from build123d import *

# Parameters (mm, degrees)
SKETCH1_R                                    = 10
BOSS_EXTRUDE1_DEPTH                          = 6
CBORE_FOR_M3_HEX_SOCKET_HEAD_CAP_SCR_2_COUNT = 2
CBORE_FOR_M3_HEX_SOCKET_HEAD_CAP_SCR_2_PITCH = 9.192388155
CBORE_FOR_M3_HEX_SOCKET_HEAD_CAP_SCR_3_COUNT = 2
CBORE_FOR_M3_HEX_SOCKET_HEAD_CAP_SCR_3_PITCH = 13
BOSS_EXTRUDE2_START                          = -6
SKETCH6_W                                    = 120
SKETCH6_H                                    = 40
SKETCH6_R                                    = 10
BOSS_EXTRUDE2_DEPTH                          = 6


# Read off the part's stored shape, not the designer's step: Tap Drill for M4 Helicoil1
with BuildPart() as part:
    # Sketch1 → Boss-Extrude1 (new body)
    with BuildSketch(Plane.XY):
        Circle(SKETCH1_R)
    extrude(amount=BOSS_EXTRUDE1_DEPTH)

    # Sketch5 → CBORE for M3 Hex Socket Head Cap Screw1 (revolve, cut)
    with BuildSketch(Plane(origin=(-6.5, 0, 6), x_dir=(0, -1, 0), z_dir=(1, 0, 0))):
        Polygon((0, 0), (0, 6), (1.7, 6), (1.7, 3.4), (3.25, 3.4), (3.25, 0.025), (3.275, 0), align=None)
    cbore_for_m3_hex_socket_head_cap_screw1 = revolve(axis=Axis((-6.5, 0, 12.35), (0, 0, -1)), mode=Mode.SUBTRACT)

    # CBORE for M3 Hex Socket Head Cap Scr 2: CBORE for M3 Hex Socket Head Cap Screw1 ×2
    with Locations(*[Vector(0.7071067811865476, 0.7071067811865476, 0) * (i * CBORE_FOR_M3_HEX_SOCKET_HEAD_CAP_SCR_2_PITCH) for i in range(1, CBORE_FOR_M3_HEX_SOCKET_HEAD_CAP_SCR_2_COUNT)]):
        add(cbore_for_m3_hex_socket_head_cap_screw1, mode=Mode.SUBTRACT)

    # CBORE for M3 Hex Socket Head Cap Scr 3: CBORE for M3 Hex Socket Head Cap Screw1 ×2
    with Locations(*[(i * CBORE_FOR_M3_HEX_SOCKET_HEAD_CAP_SCR_3_PITCH, 0, 0) for i in range(1, CBORE_FOR_M3_HEX_SOCKET_HEAD_CAP_SCR_3_COUNT)]):
        add(cbore_for_m3_hex_socket_head_cap_screw1, mode=Mode.SUBTRACT)

    # Sketch6 → Boss-Extrude2 (add)
    with BuildSketch(Plane.XY.offset(6).offset(BOSS_EXTRUDE2_START)):
        Rectangle(SKETCH6_W, SKETCH6_H)
        Circle(SKETCH6_R, mode=Mode.SUBTRACT)
    extrude(amount=BOSS_EXTRUDE2_DEPTH)

    # Tap Drill for M4 Helicoil1 outline → Tap Drill for M4 Helicoil1 (revolve, cut)
    with BuildSketch(Plane(origin=(55, -15, 0), x_dir=(1, 0, 0), z_dir=(0, -1, 0))):
        Polygon((0, 0), (2.1, 0), (2.1, 5.975), (2.125, 6), (0, 6), align=None)
    revolve(axis=Axis((55, -15, 0), (0, 0, 1)), mode=Mode.SUBTRACT)

    # Tap Drill for M4 Helicoil1 2 outline → Tap Drill for M4 Helicoil1 2 (revolve, cut)
    with BuildSketch(Plane(origin=(-55, -15, 0), x_dir=(1, 0, 0), z_dir=(0, -1, 0))):
        Polygon((0, 0), (2.1, 0), (2.1, 5.975), (2.125, 6), (0, 6), align=None)
    revolve(axis=Axis((-55, -15, 0), (0, 0, 1)), mode=Mode.SUBTRACT)

    # Tap Drill for M4 Helicoil1 3 outline → Tap Drill for M4 Helicoil1 3 (revolve, cut)
    with BuildSketch(Plane(origin=(-55, 15, 0), x_dir=(1, 0, 0), z_dir=(0, -1, 0))):
        Polygon((0, 0), (2.1, 0), (2.1, 5.975), (2.125, 6), (0, 6), align=None)
    revolve(axis=Axis((-55, 15, 0), (0, 0, 1)), mode=Mode.SUBTRACT)

    # Tap Drill for M4 Helicoil1 4 outline → Tap Drill for M4 Helicoil1 4 (revolve, cut)
    with BuildSketch(Plane(origin=(55, 15, 0), x_dir=(1, 0, 0), z_dir=(0, -1, 0))):
        Polygon((0, 0), (2.1, 0), (2.1, 5.975), (2.125, 6), (0, 6), align=None)
    revolve(axis=Axis((55, 15, 0), (0, 0, 1)), mode=Mode.SUBTRACT)


solid = part.part
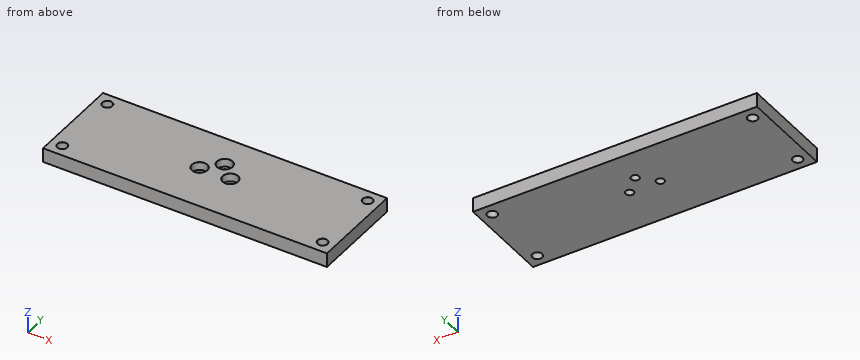
Design review of the part built by this model. Coordinates are the model's own, in mm. Round coordinates to 2 decimals unless told otherwise and drop trailing zeros. Loops run counter-clockwise (first coordinate to the right, second up) from the corner with the lowest first, then second, coordinate; pieces in that order, holes last. Notation, with made-up numbers: M -14,12 L 42,12 A17 ccw 42,37 Z; hole C 33,83 d3. An arc over 180 degrees is marked long. Answer as a JSON object with one key per item and string values.
Item 1: We need section A-A on y = 15. Give the boundary of the cut face in (x, z) (3 decimals).
Answer sheet:
{"outline": "M -60,0 L -57.1,0 L -57.1,5.975 L -57.125,6 L -60,6 Z; M -52.9,0 L 52.9,0 L 52.9,5.975 L 52.875,6 L -52.875,6 L -52.9,5.975 Z; M 57.1,0 L 60,0 L 60,6 L 57.125,6 L 57.1,5.975 Z"}
Item 2: We need section C-C on x = -55. Give the boundary of the cut face in (y, z) (3 decimals), and give its area (3 significant figures).
Answer sheet:
{"outline": "M -20,0 L -17.1,0 L -17.1,5.975 L -17.125,6 L -20,6 Z; M -12.9,0 L 12.9,0 L 12.9,5.975 L 12.875,6 L -12.875,6 L -12.9,5.975 Z; M 17.1,0 L 20,0 L 20,6 L 17.125,6 L 17.1,5.975 Z", "area": "190 mm^2"}
Item 3: We need section D-D on y = 6.5. Give the boundary of the cut face in (x, z) (3 decimals), and give its area (3 significant figures).
Answer sheet:
{"outline": "M -60,0 L -1.7,0 L -1.7,2.6 L -3.25,2.6 L -3.25,5.975 L -3.275,6 L -60,6 Z; M 1.7,0 L 60,0 L 60,6 L 3.275,6 L 3.25,5.975 L 3.25,2.6 L 1.7,2.6 Z", "area": "689 mm^2"}
Item 4: Wall thickness on L1, parallel to X at y = 0, z = 1.2; L2, parallel to Y at x = -55, z = 3.75; L3, parallel to X at y = 0, z = 4.15: over which ranges is each line inside the solid? List them lowest first. Write a range as from..to.
Answer sheet:
{"L1": "x = -60..-8.2, -4.8..4.8, 8.2..60", "L2": "y = -20..-17.1, -12.9..12.9, 17.1..20", "L3": "x = -60..-9.75, -3.25..3.25, 9.75..60"}
Item 5: We need section B-B on z = 1.6. Give the boundary of the cut face in (x, y), and give its area (3 significant figures).
Answer sheet:
{"outline": "M -60,-20 L 60,-20 L 60,20 L -60,20 Z; hole C -55,-15 d4.2; hole C -55,15 d4.2; hole C -6.5,0 d3.4; hole C 0,6.5 d3.4; hole C 6.5,0 d3.4; hole C 55,-15 d4.2; hole C 55,15 d4.2", "area": "4,720 mm^2"}
Item 6: Clearance check with flat-ended pins moving along their axes: P1, Ø3.5, axis at x = 55, y = -15, coming from the +Z side; P2, Ø5.5, axis at x = 0, y = 6.5, coming from the +Z side. State where each tip first meets the part, or that it passes through.
Answer sheet:
{"P1": "passes through", "P2": "stops at z = 2.6"}
